Design review of the part shown in the three views and the two pictorial views. Dimensions are in mm from the part's minimum x, y and z. A direction names the side the tool comes from. Round coordinates to 2 decimals unless told otherwise and drop trailing zeros. Order: outer loops, then holes, each group sorted by start corner. A loop starts at its lowest first (then second) coordinate and runs counter-clockwise, first axis right, second up. Notation, with made-up numbers: M 10.25,49.25 L 41.25,49.25 A19 cw 41.25,79.25 Z; hole C -1,-11 d2. An arc over 180 degrees is marked long. Use a Markdown table: item, result. Add a question column.
(1) Take a section at B-B (x = 10). Write out the cut boundary in (y, z).
(2) The part is to be moulded in two halves that separate along X. For the marked faces 4, 5 and 6, say which applies: released by +X, released by -X, zero draft, split by the parting line, or undercut.
(3) To check wall thickness, follow probe 1 along Z at (x, y) = (10, 10.75); probe 2 along Z at (x, y) = (10, 6.5); probe 3 along Z at (x, y) = (3.25, 3.5). State the ranges of each line that lie inside material, in increasing order. Write a range as from..to.
(4) Take a section at D-D (x = 13.5). Write out the cut boundary in (y, z).
(5) Take a section at A-A (y = 10). Write out the cut boundary in (x, z).
(6) For pin 1 (4 mm diameter, centred on x = 10.5, y = 17, fed in from -Z); pin 2 (2 mm diameter, centred on x = 4, z = 10.5, fed in from +Y); pin 3 (4 mm diameter, centred on y = 12.5, z = 16, fed in from -X), all flat-tipped, find the tip position at first contact; note any pin that passes through.
(7) Take a section at C-C (z = 12.25). Write out the cut boundary in (x, y).
(8) Machinability: for the marked faces 1, 2 and 3, which of the approach directions +Z, -Z, +X, -X, +Y, -Y give a long, thin tool a straight path to every point of the face, cutting with its end or side? Answer none if there is none.
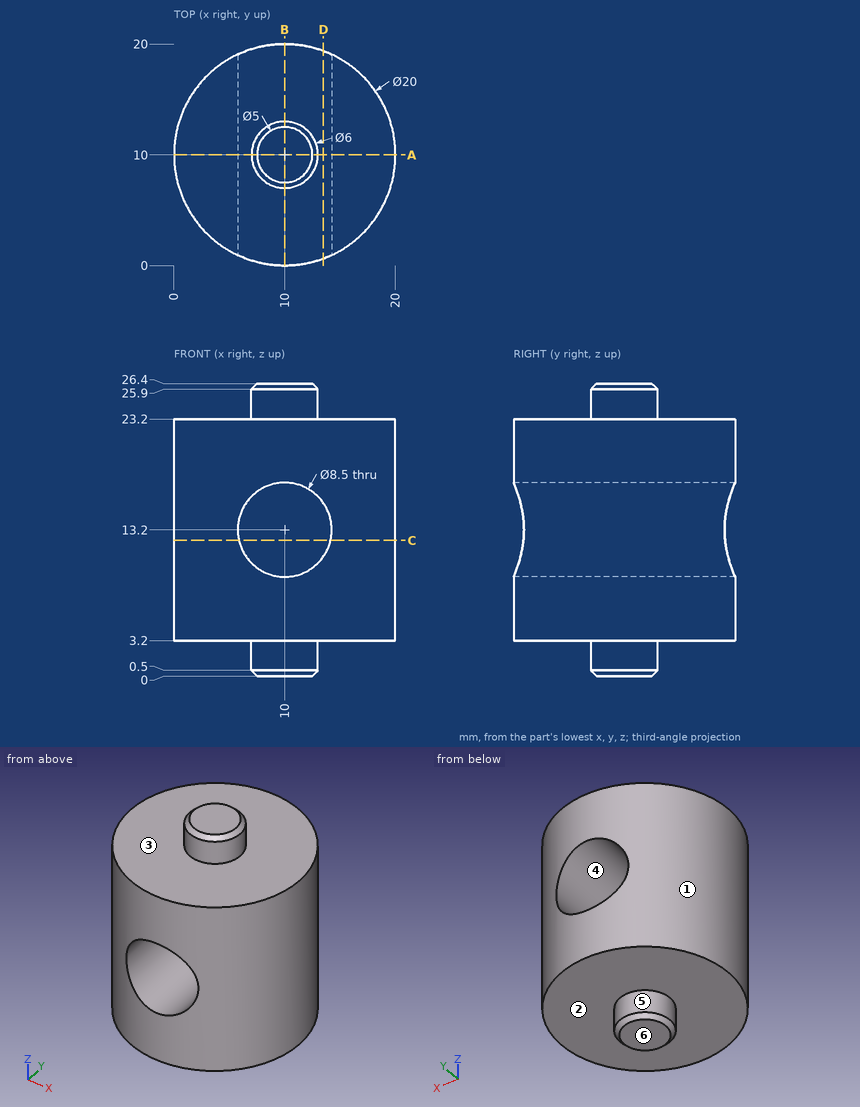
Verdict:
| question | item | result |
|---|---|---|
| 1 | outline | M 0,3.2 L 7,3.2 L 7,0.5 L 7.5,0 L 12.5,0 L 13,0.5 L 13,3.2 L 20,3.2 L 20,8.95 L 0,8.95 Z; M 0,17.45 L 20,17.45 L 20,23.2 L 13,23.2 L 13,25.9 L 12.5,26.4 L 7.5,26.4 L 7,25.9 L 7,23.2 L 0,23.2 Z |
| 2 | face 4 | undercut |
| 2 | face 5 | split by the parting line |
| 2 | face 6 | zero draft |
| 3 | probe 1 | z = 0..8.95, 17.45..26.4 |
| 3 | probe 2 | z = 3.2..8.95, 17.45..23.2 |
| 3 | probe 3 | z = 3.2..23.2 |
| 4 | outline | M 0.63,3.2 L 19.37,3.2 L 19.37,10.79 L 0.63,10.79 Z; M 0.63,15.61 L 19.37,15.61 L 19.37,23.2 L 0.63,23.2 Z |
| 5 | outline | M 0,3.2 L 7,3.2 L 7,0.5 L 7.5,0 L 12.5,0 L 13,0.5 L 13,3.2 L 20,3.2 L 20,23.2 L 13,23.2 L 13,25.9 L 12.5,26.4 L 7.5,26.4 L 7,25.9 L 7,23.2 L 0,23.2 Z; hole C 10,13.2 d8.5 |
| 6 | pin 1 | stops at z = 3.2 |
| 6 | pin 2 | stops at y = 18.66 |
| 6 | pin 3 | stops at x = 0.01 |
| 7 | outline | M 5.86,0.9 L 5.86,19.1 A10 ccw Z; M 14.14,0.9 A10 ccw 14.14,19.1 Z |
| 8 | face 1 | +Z, -Z |
| 8 | face 2 | -Z |
| 8 | face 3 | +Z |
